Autodesk Inventor part; units mm, degrees
ref_plane "YZ Plane" through (0, 0, 0) normal (1, 0, 0) x (0, 1, 0)
ref_plane "XZ Plane" through (0, 0, 0) normal (0, 1, 0) x (-1, 0, 0)
ref_plane "XY Plane" through (0, 0, 0) normal (0, 0, 1) x (1, 0, 0)
sketch "Sketch1" plane through (0, 0, 0) normal (0, 1, 0) x (-1, 0, 0)
  line L0 (-10, -1.5) -> (10, -1.5)
  line L1 (10, 3.5) -> (10, 3.5)
  line L2 (10, 1.5) -> (-10, 1.5)
  line L3 (-10, 3.5) -> (-10, 3.5)
  line L4 (-10, -1.5) -> (10, 1.5) construction
  line L5 (10, -1.5) -> (-10, 1.5) construction
  circle A0 centre (8.5, 0) radius 1
  line L6 (-10, 1.5) -> (-10, -1.5)
  line L7 (10, 1.5) -> (10, -1.5)
  line L8 (-10, 1.5) -> (-4, 1.5)
  circle A1 centre (-8.5, 0) radius 1
  point P0 (0, 0)
  dimension "d0" = 3
  dimension "d1" = 20
  dimension "d3" = 2
  dimension "d6" = 1.5
  dimension "d8" = 1.5
  dimension "d21" = 2
  dimension "d22" = 1.5
  dimension "d23" = 1.5
extrude "Extrusion1" add sketch "Sketch1" along normal blind 5
properties part number "link"
Check sheet for the modelled part. Datum: model origin and axes. Units: mm. Give positions to 0.01 mm unless a question says otherwise; leave off trailing zeros. Write each loop counter-clockwise with the first axis right and the second up, starting at its lowest first coordinate (ties: lowest second). Pieces come first, ordered by that corner, then holes. Notation, with made-up numbers: (89.25, 49) - (98.25, 49) arc R15 ccw to (98.25, 75) - close; hole circle Ø2 at (87, -1.75). An arc over 180 degrees is marked (long way). Answer as a JSON object with one key per item and string values. Group by question number.
1) Sectioned sample at C-C (y = 2.1). Record the cut outline in (x, z).
2) Thickness scan on probe 1 along Z at (x, y) = (-8.5, 1.3); probe 2 along X at (y, z) = (3.3, 0.75); probe 3 along X at (y, z) = (2.4, 0.9). Record the ranges inside material, lowest first. Write a range as from..to.
3) Release check for a two-part mould opening along Z. For faces 1 (the face through (-10, 2, 0)), 2 (the face through (9.3, 2.5, 0.6)), 3 (the face through (0, 2, -1.5)) record: pulls with the +Z half, pulls with the -Z half, needs draft (parallel to the pull), parting line crosses it, or undercut.
4) Depth check by flat-ended pin: P1, Ø1.2, axis at x = 8.5, z = 0, coming from the +Y side; P2, Ø1, axis at x = 6, z = 0, coming from the -Y side. Enter the tip coordinate at first touch or a pass-through.
5) Sectioned sample at B-B (z = 0). Record the cut outline in (x, y).
6) Sectioned sample at A-A (x = -8.5). Record the cut outline in (y, z).
Geometry results:
{
 "1": {"outline": "(-10, -1.5) - (10, -1.5) - (10, 1.5) - (-10, 1.5) - close; hole circle Ø2 at (-8.5, 0); hole circle Ø2 at (8.5, 0)"},
 "2": {"probe 1": "z = -1.5..-1, 1..1.5", "probe 2": "x = -10..-9.16, -7.84..7.84, 9.16..10", "probe 3": "x = -10..-8.94, -8.06..8.06, 8.94..10"},
 "3": {"face 1": "needs draft", "face 2": "undercut", "face 3": "pulls with the -Z half"},
 "4": {"P1": "passes through", "P2": "stops at y = 0"},
 "5": {"outline": "(-10, 0) - (-9.5, 0) - (-9.5, 5) - (-10, 5) - close; (-7.5, 0) - (7.5, 0) - (7.5, 5) - (-7.5, 5) - close; (9.5, 0) - (10, 0) - (10, 5) - (9.5, 5) - close"},
 "6": {"outline": "(0, -1.5) - (5, -1.5) - (5, -1) - (0, -1) - close; (0, 1) - (5, 1) - (5, 1.5) - (0, 1.5) - close"}
}
